The listing builds one solid part. Answer for the finished solid, in the listing's coordinates (mm). Face numbers are marked on the shaded views. A direction names the side the tool comes from. Give positions to 0.01 mm unless a question says otherwise; leave off trailing zeros. Write each loop counter-clockwise with the first axis right and the second up, starting at its lowest first coordinate (ties: lowest second). Pieces come first, ordered by that corner, then holes.
Autodesk Inventor part; units mm, degrees
ref_plane "YZ Plane" through (0, 0, 0) normal (1, 0, 0) x (0, 1, 0)
ref_plane "XZ Plane" through (0, 0, 0) normal (0, 1, 0) x (-1, 0, 0)
ref_plane "XY Plane" through (0, 0, 0) normal (0, 0, 1) x (1, 0, 0)
ref_plane "Work Plane1" through (0, 0, 0) normal (0, 0, 1) x (1, 0, 0)
sketch "Sketch1" plane through (0, 0, 0) normal (0, 0, 1) x (1, 0, 0)
  circle A0 centre (-15, -15) radius 1.2
  circle A1 centre (-89, -15) radius 1.2
  circle A2 centre (-89, -15) radius 1.75
  line L0 (-89, -15) -> (-112.137643, -5.443064) construction
  line L1 (-87.137402, -10.359731) -> (-91.777544, -8.497184)
  line L2 (-95.50274, -17.777722) -> (-90.862598, -19.640269)
  arc A3 (-90.862598, -19.640269) -> (-87.137402, -10.359731) centre (-89, -15) ccw
  line L3 (-95.50274, -17.777722) -> (-91.777544, -8.497184)
  point P0 (-100.568822, -10.221532)
  dimension "d1" = 3.5
  dimension "d10" = 5
extrude "Extrusion1" add sketch "Sketch1" along normal blind 10 contours A3 L2 L3 L1
ref_plane "Work Plane2" through (-109.423166, -12.19008, 0) normal (-0.9280284, 0.3725094, 0) x (0, 0, 1)
sketch "Sketch3" plane through (-109.423166, -12.19008, 0) normal (-0.9280284, 0.3725094, 0) x (0, 0, 1)
  line L0 (0, 10.000274) -> (0, 0)
  line L1 (0, 0) -> (10, 0)
  line L2 (10, 10.000274) -> (10, 0)
  line L3 (0, 10.000274) -> (10, 10.000274)
  circle A0 centre (4.999863, 5.000137) radius 5.000137
  point P0 (0, 52.073903)
sketch "Sketch3 outline for Loft1" plane through (-109.423166, -12.19008, 0) normal (-0.9280284, 0.3725094, 0) x (0, 0, 1)
  circle A0 centre (4.999863, 5.000137) radius 5.000137
loft "Loft1" add profiles "Sketch3 outline for Loft1" section 2 edges at (-93.640142, -13.137453, 0) (-95.50274, -17.777722, 5) (-93.640142, -13.137453, 10) (-91.777544, -8.497184, 5)
sketch "Sketch5" plane through (0, 0, 10) normal (0, 0, 1) x (1, 0, 0)
  circle A0 centre (-89, -15) radius 5.25
  arc A1 (-90.862598, -19.640269) -> (-87.137402, -10.359731) centre (-89, -15) ccw
  point P0 (0, 0)
  dimension "d18" = 10.5
extrude "Extrusion3" cut sketch "Sketch5" against normal blind 5
sketch "Sketch6" plane through (0, 0, 10) normal (0, 0, 1) x (1, 0, 0)
  line L0 (-99.397863, -14.059118) -> (-102.181949, -12.94159)
  line L1 (-102.181949, -12.94159) -> (-99.946892, -7.373419)
  line L2 (-99.946892, -7.373419) -> (-97.162807, -8.490948)
  line L3 (-97.162807, -8.490948) -> (-99.397863, -14.059118)
  line L4 (-116.544319, -29.930925) -> (-85.605283, 47.147132)
  line L5 (-95.50274, -17.777722) -> (-92.347771, -19.044123)
  point P0 (0, 0)
  dimension "d21" = 7
  dimension "d22" = 3
  dimension "d23" = 6
  dimension "d24" = 2
extrude "Extrusion4" cut sketch "Sketch6" against normal blind 9
sketch "Sketch7" plane through (-107.560568, -7.549811, 4.999863) normal (-0.9280284, 0.3725094, 0) x (0, 0, 1)
  arc A0 (-3.535582, -3.535679) -> (3.535582, -3.535679) centre (0, 0) ccw
  point P0 (-4.999863, 47.073766)
hole "Hole1" at (-107.560568, -7.549811, 4.999863) direction (0.9280284, -0.3725094, 0) diameter 3.5 depth 7
sketch "Sketch8" plane through (0, 0, 10) normal (0, 0, 1) x (1, 0, 0)
  line L0 (-88.622575, -9.763584) -> (-91.777544, -8.497184)
  arc A0 (-88.622575, -9.763584) -> (-93.043836, -11.651883) centre (-89, -15) ccw
  spline S0 degree 2 poles (-93.872149, -13.044325) (-93.566724, -12.283424) (-93.043836, -11.651883) knots 0 0 0 1 1 1 weights 1 0.98802352 1
  line L1 (-93.872149, -13.044325) -> (-92.009551, -8.404056)
  arc A1 (-88.622575, -9.763584) -> (-92.347771, -19.044123) centre (-89, -15) ccw
  line L2 (-92.009551, -8.404056) -> (-88.622575, -9.763584)
  point P0 (0, 0)
extrude "Extrusion5" cut sketch "Sketch8" against normal blind 5
properties part number "Hangar"
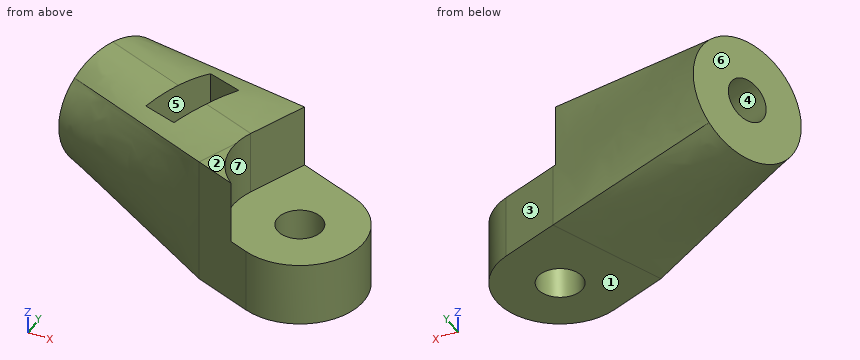
Item 1: A cutting plane is placed at B-B, the plane x = -86. Give the vertices of the cut face in (y, z), plus the area to 3 significant figures.
Conclusion:
outline: (-19, 0) - (-11, 0) - (-11, 5) - (-19, 5) - close
area: 40.0 mm2
Item 2: Each of these flat-tipped pins is pushed along its axis until it touches: P1, Ø8, axis at x = -88, y = -12, coming from the +Z side; P2, Ø1, axis at y = -5, z = 2, coming from the -X side; P3, Ø4, axis at y = -7.5, z = 7, coming from the +X side. Where does it stop, or does it pass through?
Conclusion:
P1: stops at z = 5
P2: stops at x = -106.74
P3: stops at x = -92.01
Item 3: Determine the mould class of the marked faces 1, 2, 3 and 4 for opening direction Z: pulls with the +Z half, pulls with the -Z half, needs draft (parallel to the pull), parting line crosses it, or undercut.
Conclusion:
face 1: pulls with the -Z half
face 2: pulls with the +Z half
face 3: needs draft
face 4: undercut
Item 4: Which of the six approach directions +Z, -Z, +X, -X, +Y, -Y give full straight-line access (tool end or side, diameter ignored) to the marked faces 5, 6 and 7?
Conclusion:
face 5: +Z
face 6: +Z, -Z, -X, +Y
face 7: +Z, +X
Item 5: A cutting plane is placed at A-A, the plane x = -89. Give the vertices of the cut face in (y, z).
Conclusion:
outline: (-20, 0) - (-16.75, 0) - (-16.75, 5) - (-20, 5) - close; (-13.25, 0) - (-9.61, 0) - (-9.61, 5) - (-13.25, 5) - close
Item 6: Consider probe 1 along X at (y, z) = (-12.5, 3.25); probe 2 along X at (y, z) = (-15, 1.5); probe 3 along Y at (x, z) = (-89, 2.1). Determine where each line is inside the solid, lowest interval first.
Conclusion:
probe 1: x = -107.93 to -102, -98.77 to -84.67
probe 2: x = -101.35 to -90.75, -87.25 to -84
probe 3: y = -20 to -16.75, -13.25 to -9.61
